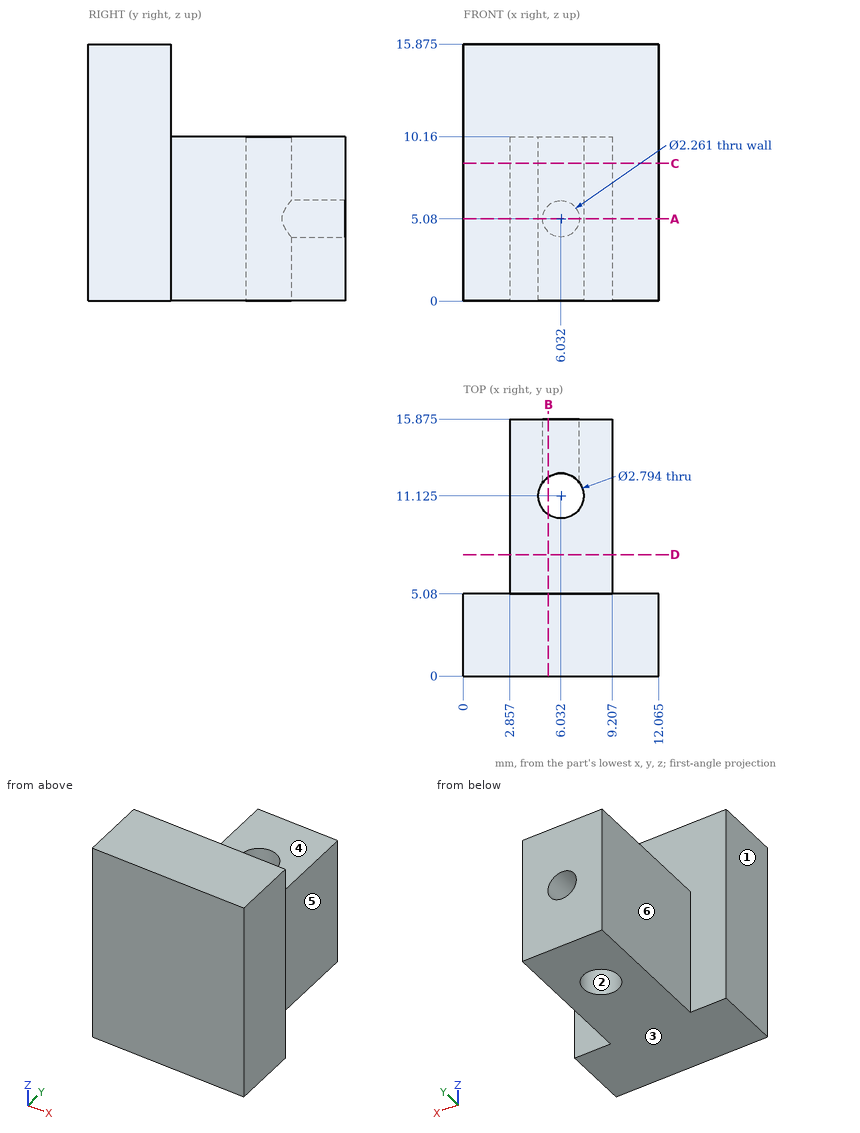
Design review of the part shown in the three views and the two pictorial views. Dimensions are in mm from the part's minimum x, y and z. A direction names the side the tool comes from. Give positions to 0.01 mm unless a question says otherwise; leave off trailing zeros. Write each loop counter-clockwise with the first axis right and the second up, starting at its lowest first coordinate (ties: lowest second). Pieces come first, ordered by that corner, then holes.
Item 1: Wall thickness on probe 1 along X at (y, z) = (14.5, 5.08); probe 2 along Z at (x, y) = (6.25, 9); probe 3 along Y at (x, z) = (10, 1.75): over which ranges is each line inside the solid? List them lowest first.
Item 2: Take a section at A-A (z = 5.08). Give the boundary of the cut face in (x, y) (1 decimal), and give its area (3 significant figures).
Item 3: Take a section at D-D (y = 7.5). Give the boundary of the cut face in (x, z), and give its area (3 significant figures).
Item 4: Take a section at C-C (z = 8.5). Give the boundary of the cut face in (x, y) (1 decimal).
Item 5: Take a section at B-B (x = 5.25). Give the boundary of the cut face in (y, z) (1 decimal), and give its area (3 significant figures).
Item 6: Insertion check: P1, Ø7, axis at x = 6.5, y = 9.5, coming from the +Z side; P2, Ø5, axis at y = 9.5, z = 5, coming from the +X side; P3, Ø8, axis at y = 13, z = 6, coming from the -X side. Each pin has a flat end and moves straight along its axis. Give the tip position at first contact, or say it passes through.
Item 7: The part is to be moulded in two halves that separate along X. For the marked faces 1, 2 and 3, say which applies: +X half, -X half, draft (parallel to the pull), parting line (faces both ways), or undercut.
Item 8: Machinability: for the marked faces 4, 5 and 6, which of the approach directions +Z, -Z, +X, -X, +Y, -Y give a long, thin tool a straight path to every point of the face, cutting with its end or side? Answer none if there is none.
Established:
1. probe 1: x = 2.86 to 4.9, 7.16 to 9.21
1. probe 2: z = 0 to 10.16
1. probe 3: y = 0 to 5.08
2. outline: (0, 0) - (12.1, 0) - (12.1, 5.1) - (9.2, 5.1) - (9.2, 15.9) - (7.2, 15.9) - (7.2, 11.9) arc R1.4 cw (long way) to (4.9, 11.9) - (4.9, 15.9) - (2.9, 15.9) - (2.9, 5.1) - (0, 5.1) - close
2. area: 116 mm2
3. outline: (2.86, 0) - (9.21, 0) - (9.21, 10.16) - (2.86, 10.16) - close
3. area: 64.5 mm2
4. outline: (0, 0) - (12.1, 0) - (12.1, 5.1) - (9.2, 5.1) - (9.2, 15.9) - (2.9, 15.9) - (2.9, 5.1) - (0, 5.1) - close; hole circle Ø2.8 at (6, 11.1)
5. outline: (0, 0) - (10, 0) - (10, 10.2) - (5.1, 10.2) - (5.1, 15.9) - (0, 15.9) - close; (12.3, 0) - (15.9, 0) - (15.9, 4.3) - (12.3, 4.3) - close; (12.3, 5.9) - (15.9, 5.9) - (15.9, 10.2) - (12.3, 10.2) - close
5. area: 161 mm2
6. P1: stops at z = 10.16
6. P2: stops at x = 9.21
6. P3: stops at x = 2.86
7. face 1: -X half
7. face 2: undercut
7. face 3: draft
8. face 4: +Z, +X, -X, +Y
8. face 5: +Z, -Z, +X, +Y
8. face 6: +Z, -Z, -X, +Y
